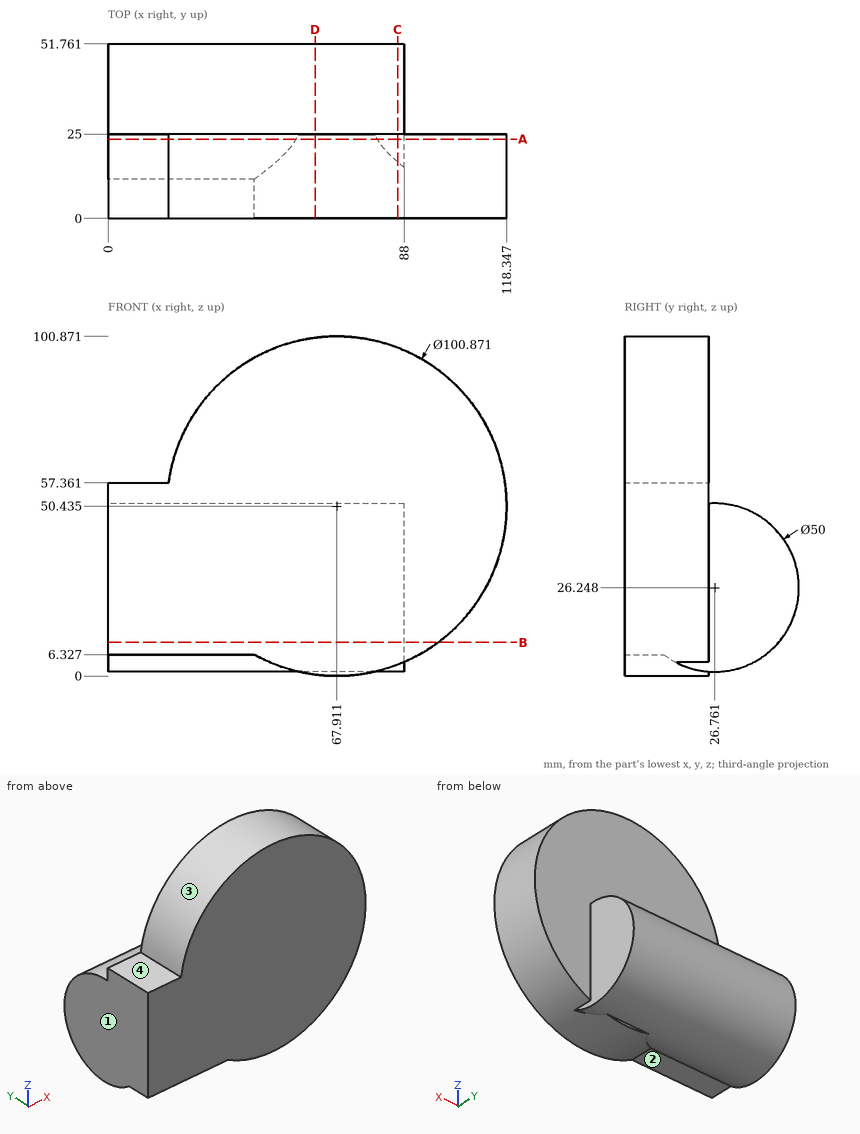
Print and shaded views of the part. All mm, measured from the part's lowest x, y and z. A direction names the side the tool comes from. Give positions to 0.01 mm unless a question says otherwise; leave off trailing zeros. Order: outer loops, then holes, each group sorted by start corner. A loop starts at its lowest first (then second) coordinate and runs counter-clockwise, first axis right, second up. Notation, with made-up numbers: (-20.75, -14.75) -> (-13.75, -14.75) arc R17 cw to (-13.75, 15.25) -> close; hole circle Ø9 at (40.5, 53). An arc over 180 degrees is marked (long way). Use CSV: the item, a comma, the result in double quotes.
1. Band-saw the part on A-A, the plane y = 23.5. Give the cut face in (x, z) (1 decimal), then the cut area to 3 significant figures.
Outcome:
outline,"(0, 1.5) -> (55.9, 1.5) arc R50.4 ccw to (80, 1.5) -> (88, 1.5) -> (88, 4.2) arc R50.4 ccw (long way) to (18, 57.4) -> (0, 57.4) -> close"
area,"9,460 mm²"
2. Band-saw the part on B-B, the plane z = 10. Give the cut face in (x, y), then the cut area to 3 significant figures.
Outcome:
outline,"(0, 0) -> (98.06, 0) -> (98.06, 25) -> (88, 25) -> (88, 45.76) -> (0, 45.76) -> close"
area,"4,280 mm²"
3. Band-saw the part on C-C, the plane x = 86. Give the cut face in (y, z) (1 decimal), then the cut area to 3 significant figures.
Outcome:
outline,"(0, 3.4) -> (16.7, 3.4) arc R25 ccw (long way) to (25, 51.2) -> (25, 97.5) -> (0, 97.5) -> close"
area,"3,430 mm²"
4. Drill centre lines: line 1 along Z through (x, y) = (17, 4.5); line 2 along Y through (x, z) = (16, 25); line 3 along X through (y, z) = (30.5, 44.5). Where is each one in solid material? Low to high. Write a range as from..to.
Outcome:
line 1,"6.33..57.36"
line 2,"0..51.73"
line 3,"0..88"
5. Band-saw the part on D-D, the plane x = 61.5. Give the cut face in (y, z), then the cut area to 3 significant figures.
Outcome:
outline,"(0, 0.41) -> (25, 0.41) -> (25, 1.31) arc R25 ccw (long way) to (25, 51.19) -> (25, 100.46) -> (0, 100.46) -> close"
area,"3,570 mm²"
6. 3-axis set-ups, long thin cutter, end or side, ignore diameter. For the marked faces 1, 2, 3 and 4: which of +Z, -Z, +X, -X, +Y, -Y reach the whole face in a straight line?
Outcome:
face 1,"+Z, -Z, -X, +Y, -Y"
face 2,"-Z, -X, -Y"
face 3,"-Y"
face 4,"+Z, -X, +Y, -Y"
7. Drop flat-ended pins along their axis: pin 1 (3.5 mm diameter, centred on x = 20, y = 3, fed in from -Z); pin 2 (1.5 mm diameter, centred on x = 47, z = 87.5, fed in from +Y); pin 3 (2 mm diameter, centred on x = 41.5, y = 33.5, fed in from +Z). Give the stop position or say it passes through.
Outcome:
pin 1,"z = 6.33"
pin 2,"y = 25"
pin 3,"z = 50.58"
